Part model, mm, in its own coordinate system. Face numbers are marked on the shaded views. A direction names the side the tool comes from. Coordinates: 2 decimals unless noted, no trailing zeros. Write each loop counter-clockwise with the first axis right and the second up, starting at its lowest first coordinate (ties: lowest second). Pieces come first, ordered by that corner, then holes. Notation, with made-up numbers: (60.25, 68.5) -> (107.25, 68.5) arc R21 cw to (107.25, 98.5) -> close; hole circle Ø1 at (57.5, -0.75). An arc over 180 degrees is marked (long way). One line per question, with ' | ' between items. Start each with the question number.
Item 1: Saw through at C-C (z = 63). List the corners of the cut face in (x, y), and give its area (3 significant figures).
Item 2: Saw through at B-B (y = -17). List the corners of the cut face in (x, z), and give its area (3 significant figures).
Item 3: Probe probe 1 along Z at (x, y) = (0, -1.9); probe 2 along X at (y, z) = (-23.5, 13.5); probe 3 along Z at (x, y) = (-58, -62). List the from-to ranges inside material, lowest first. Write a range as [from, to].
Item 4: Pin check, flat tip, straight feed: pin 1 (3.5 mm diameter, centred on x = -15, z = -15, fed in from -Y). Stop position of the tip, or through.
Item 5: Saw through at D-D (x = -11.5). List the corners of the cut face in (y, z), and give its area (3 significant figures).
Item 6: Saw through at A-A (z = 0). List the corners of the cut face in (x, y), and give its area (3 significant figures).
Item 7: 3-axis set-ups, long thin cutter, end or side, ignore diameter. For the marked faces 4 and 5: which of +Z, -Z, +X, -X, +Y, -Y reach the whole face in a straight line?
Item 8: Two-plate mould, pull along Y, no slides. Class the marked faces 1, 2 and 3: pulls with the +Y half, pulls with the -Y half, needs draft (parallel to the pull), parting line crosses it, or undercut.
from build123d import *

# Parameters (mm, degrees)
F0_W      = 120
F0_H      = 150
F1_DEPTH  = 5
F2_W      = 5
F2_H      = 150
F3_DEPTH  = 65
F4_W      = 3
F4_H      = 150
F5_DEPTH  = 10
F6_W      = 3
F6_H      = 150
F7_DEPTH  = 10
F9_DEPTH  = 150
F10_DEPTH = 150
F12_D     = 3
F13_D     = 30
F15_D     = 3


with BuildPart() as f1:
    # F0 (on Front) → F1 (new body)
    with BuildSketch(Plane.XZ):
        Rectangle(F0_W, F0_H)
    extrude(amount=F1_DEPTH)

    # F2 (on face) → F3 (join)
    with BuildSketch(Plane.XZ.offset(5)):
        with Locations((-57.5, 0)):
            Rectangle(F2_W, F2_H)
        with Locations((57.5, 0)):
            Rectangle(F2_W, F2_H)
    extrude(amount=F3_DEPTH)

    # F4 (on face) → F5 (join)
    with BuildSketch(Plane(origin=(55, 0, 0), x_dir=(0, -1, 0), z_dir=(-1, 0, 0))):
        with Locations((53.5, 0)):
            Rectangle(F4_W, F4_H)
    extrude(amount=F5_DEPTH)

    # F6 (on face) → F7 (join)
    with BuildSketch(Plane.YZ.offset(-55)):
        with Locations((-53.5, 0)):
            Rectangle(F6_W, F6_H)
    extrude(amount=F7_DEPTH)

    # F8 (on face) → F9 (join)
    with BuildSketch(Plane.XY.offset(75)):
        Polygon((55, -40.81966), (45, -52), (55, -52), align=None)
    extrude(amount=-F9_DEPTH)

    # F8 (on face) → F10 (join)
    with BuildSketch(Plane.XY.offset(75)):
        Polygon((55, -40.81966), (45, -52), (55, -52), align=None)
        Polygon((-55, -52), (-45, -52), (-55, -40.81966), align=None)
    extrude(amount=-F10_DEPTH)

    # F12 (through all)
    with Locations(Plane.XZ.offset(5)):
        with Locations((-15, 15), (0, 0), (-15, -15), (15, -15), (15, 15)):
            Hole(F12_D / 2)

    # F13 (through all)
    with Locations(Plane(origin=(0, 0, 0), x_dir=(1, 0, 0), z_dir=(0, 1, 0))):
        with Locations((0, 0)):
            Hole(F13_D / 2)

    # F15 (through all)
    with Locations(Plane.YZ.offset(60)):
        with Locations((-62.5, -67.5), (-62.5, 67.5)):
            Hole(F15_D / 2)


solid = f1.part
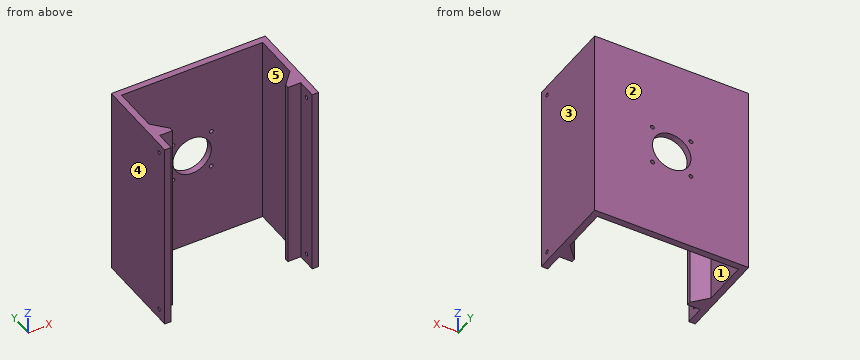
From the geometry:
1) outline: (-60, -70) -> (-55, -70) -> (-55, -55) -> (-45, -55) -> (-45, -52) -> (-55, -40.82) -> (-55, -5) -> (55, -5) -> (55, -40.82) -> (45, -52) -> (45, -55) -> (55, -55) -> (55, -70) -> (60, -70) -> (60, 0) -> (-60, 0) -> close | area: 1,420 mm2
2) outline: (-60, -75) -> (-55, -75) -> (-55, 75) -> (-60, 75) -> close; (55, -75) -> (60, -75) -> (60, 75) -> (55, 75) -> close | area: 1,500 mm2
3) probe 1: [-75, -15], [15, 75] | probe 2: [-60, -55], [55, 60] | probe 3: [-75, -68.91], [-66.09, 66.09], [68.91, 75]
4) pin 1: y = -5
5) outline: (-5, -75) -> (0, -75) -> (0, -9.63) -> (-5, -9.63) -> close; (-5, 9.63) -> (0, 9.63) -> (0, 75) -> (-5, 75) -> close | area: 654 mm2
6) outline: (-60, -70) -> (-55, -70) -> (-55, -55) -> (-45, -55) -> (-45, -52) -> (-55, -40.82) -> (-55, -5) -> (-15, -5) -> (-15, 0) -> (-60, 0) -> close; (15, -5) -> (55, -5) -> (55, -40.82) -> (45, -52) -> (45, -55) -> (55, -55) -> (55, -70) -> (60, -70) -> (60, 0) -> (15, 0) -> close | area: 1,270 mm2
7) face 4: +Z, -Z, -X, +Y, -Y | face 5: +Z, -Z
8) face 1: undercut | face 2: pulls with the +Y half | face 3: needs draft
